```python
from build123d import *

# Parameters (mm, degrees)
F0_W     = 20
F0_H     = 6
F0_W_2   = 9
F0_H_2   = 20
F1_DEPTH = 6
F2_DEPTH = 6
F3_R     = 2.25
F3_R_2   = 1.143
F4_DEPTH = 3
F5_DEPTH = 6.001


with BuildPart() as f1:
    # F0 (on Right) → F1 (new body)
    with BuildSketch(Plane.YZ):
        Polygon((-36, -10), (-36, -36), (-10, -36), (-10, -30), (10, -30), (10, -36), (36, -36), (36, -10), (27, -10), (27, 10), (36, 10), (36, 36), (10, 36), (10, 30), (-10, 30), (-10, 36), (-36, 36), (-36, 10), (-27, 10), (-27, -10), align=None)
        with Locations((0, -33)):
            Rectangle(F0_W, F0_H)
        with Locations((-31.5, 0)):
            Rectangle(F0_W_2, F0_H_2)
        with Locations((31.5, 0)):
            Rectangle(F0_W_2, F0_H_2)
        with Locations((0, 33)):
            Rectangle(F0_W, F0_H)
    extrude(amount=F1_DEPTH)

    # F0 (on Right) → F2 (cut, through all)
    with BuildSketch(Plane.YZ):
        with Locations((0, 33)):
            Rectangle(F0_W, F0_H)
        with Locations((31.5, 0)):
            Rectangle(F0_W_2, F0_H_2)
        with Locations((0, -33)):
            Rectangle(F0_W, F0_H)
        with Locations((-31.5, 0)):
            Rectangle(F0_W_2, F0_H_2)
    extrude(amount=F2_DEPTH, mode=Mode.SUBTRACT)

    # F3 (on face) → F4 (cut)
    with BuildSketch(Plane.YZ.offset(6)):
        with Locations((-33, 20.857)):
            Circle(F3_R)
        with Locations((-33, 20.857)):
            Circle(F3_R_2, mode=Mode.SUBTRACT)
        with Locations((-33, -20.857)):
            Circle(F3_R)
        with Locations((-33, -20.857)):
            Circle(F3_R_2, mode=Mode.SUBTRACT)
        with Locations((33, 20.857)):
            Circle(F3_R)
        with Locations((33, 20.857)):
            Circle(F3_R_2, mode=Mode.SUBTRACT)
        with Locations((33, -20.857)):
            Circle(F3_R)
        with Locations((33, -20.857)):
            Circle(F3_R_2, mode=Mode.SUBTRACT)
    extrude(amount=-F4_DEPTH, mode=Mode.SUBTRACT)

    # F5 (cut, through all): faces of the model
    f5_faces = [f1.faces().sort_by_distance(p)[0] for p in [
        (6, -33, 20.857),
        (6, 33, 20.857),
        (6, 33, -20.857),
        (6, -33, -20.857),
    ]]
    extrude(f5_faces, amount=-F5_DEPTH, mode=Mode.SUBTRACT)


solid = f1.part
```
Could you check a few things on this model? Use its own coordinates, in mm. A direction names the side the tool comes from. Round coordinates to 2 decimals unless told otherwise and drop trailing zeros. Order: outer loops, then holes, each group sorted by start corner. A loop starts at its lowest first (then second) coordinate and runs counter-clockwise, first axis right, second up. Notation, with made-up numbers: M 62,12.25 L 95,12.25 A27 ccw 95,30.25 Z; hole C -5,-20.75 d2. An arc over 180 degrees is marked long. One line per question, with ' | ' between items. Start each with the question number.
(1) Suppose I cut it at B-B on z = -31. List the corners of the cut face in (x, y) for me.
(2) Suppose I cut it at C-C on x = 4.6. List the corners of the cut face in (y, z) for me.
(3) For faces 4 (the face through (3, 0, 30)), 5 (the face through (3, -34, -20)), 6 (the face through (3, 31, 10)), which set-ups out of +Z, -Z, +X, -X, +Y, -Y let a thin tool reach every point of the face, with its end or its side?
(4) For P1, Ø3.5, axis at y = -33, z = -20.857, coming from the +X side; P2, Ø3, axis at x = 2.5, z = 0, coming from the -Y side, each with a flat end and sliding along its axis, tell me the tip position at first contact or that it passes through.
(5) Please list where these lines run through material, in increasing order: line 1 along Z through (x, y) = (5, -33); line 2 along Z through (x, y) = (1, -33); line 3 along Y through (x, z) = (1.95, -31.5).
(6) Suppose I cut it at A-A on y = 33. List the corners of the cut face in (x, z) for me, then the cut area to 3 significant figures.
(7) Suppose I cut it at D-D on y = -9. List the corners of the cut face in (x, z) for me.
(8) Thinking about a two-plate mould opening in Y: for faces 1 (the face through (3, -36, 23)), 2 (the face through (1.52, 31.86, 20.91)), 3 (the face through (3, -23, 36)), which applies, +Y half, -Y half, draft (parallel to the pull), parting line (faces both ways), or undercut?
Geometry results:
1) outline: M 0,-36 L 6,-36 L 6,-10 L 0,-10 Z; M 0,10 L 6,10 L 6,36 L 0,36 Z
2) outline: M -36,-36 L -10,-36 L -10,-30 L 10,-30 L 10,-36 L 36,-36 L 36,-10 L 27,-10 L 27,10 L 36,10 L 36,36 L 10,36 L 10,30 L -10,30 L -10,36 L -36,36 L -36,10 L -27,10 L -27,-10 L -36,-10 Z; hole C -33,-20.86 d4.5; hole C -33,20.86 d4.5; hole C 33,-20.86 d4.5; hole C 33,20.86 d4.5
3) face 4: +Z, +X, -X | face 5: +X | face 6: +X, -X, +Y
4) P1: x = 3 | P2: y = -27
5) line 1: -36 to -23.11, -18.61 to -10, 10 to 18.61, 23.11 to 36 | line 2: -36 to -22, -19.71 to -10, 10 to 19.71, 22 to 36 | line 3: -36 to -10, 10 to 36
6) outline: M 0,-36 L 6,-36 L 6,-23.11 L 3,-23.11 L 3,-22 L 0,-22 Z; M 0,-19.71 L 3,-19.71 L 3,-18.61 L 6,-18.61 L 6,-10 L 0,-10 Z; M 0,10 L 6,10 L 6,18.61 L 3,18.61 L 3,19.71 L 0,19.71 Z; M 0,22 L 3,22 L 3,23.11 L 6,23.11 L 6,36 L 0,36 Z | area: 271 mm²
7) outline: M 0,-30 L 6,-30 L 6,30 L 0,30 Z
8) face 1: -Y half | face 2: undercut | face 3: draft
